Verification items for this drawing (mm, ordinates from the low corner). A direction names the side the tool comes from. Round coordinates to 2 decimals unless told otherwise and drop trailing zeros. Loops run counter-clockwise (first coordinate to the right, second up) from the corner with the lowest first, then second, coordinate; pieces in that order, holes last. Notation, with made-up numbers: (75.5, -27) - (121.5, -27) arc R28 cw to (121.5, -5) - close; hole circle Ø3 at (4.25, 19). An arc over 180 degrees is marked (long way). Put each result on its own line as item: value.
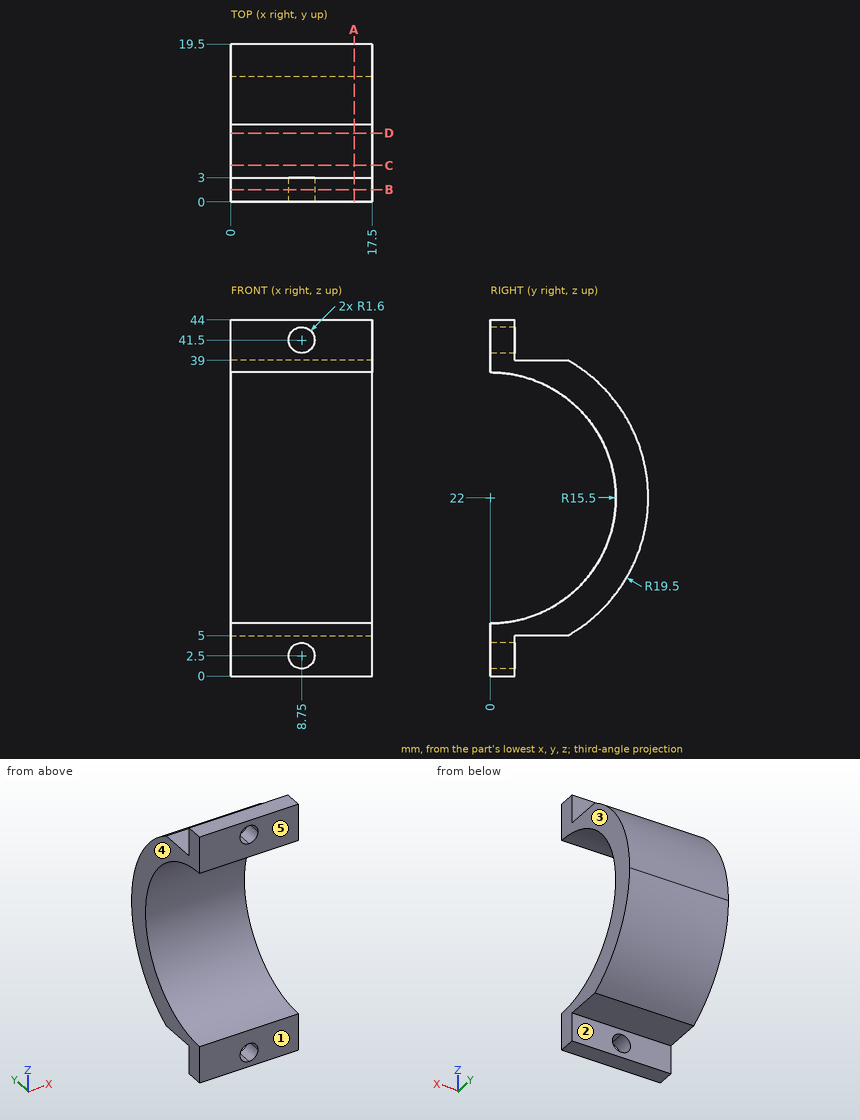
Item 1: Section check D-D on y = 8.5. Enter the section's corners in (x, z), then the cut area to 3 significant figures.
Filled sheet:
outline: (0, 5) - (17.5, 5) - (17.5, 9.04) - (0, 9.04) - close; (0, 34.96) - (17.5, 34.96) - (17.5, 39) - (0, 39) - close
area: 141 mm²
Item 2: Section check B-B on y = 1.5. Enter the section's corners in (x, z), then the cut area to 3 significant figures.
Filled sheet:
outline: (0, 0) - (17.5, 0) - (17.5, 6.57) - (0, 6.57) - close; (0, 37.43) - (17.5, 37.43) - (17.5, 44) - (0, 44) - close; hole circle Ø3.2 at (8.75, 2.5); hole circle Ø3.2 at (8.75, 41.5)
area: 214 mm²
Item 3: Thickness scan on line 1 (Y direction, x = 5, z = 4); line 2 (Z direction, x = 5.75, y = 3.5); line 3 (Y direction, x = 13, z = 22). Record the ranges inside material, lowest first. Write a range as from..to.
Filled sheet:
line 1: 0..3
line 2: 5..6.9, 37.1..39
line 3: 15.5..19.5
Item 4: Go/stop test with flat-tipped pins: pin 1 (2.5 mm diameter, centred on x = 10.5, z = 2, fed in from +Y); pin 2 (2 mm diameter, centred on x = 7, y = 14, fed in from -Z); pin 3 (5 mm diameter, centred on x = 10.5, y = 7, fed in from +Z). Record where each tip stops, or that it passes through.
Filled sheet:
pin 1: y = 3
pin 2: z = 7.47
pin 3: z = 39
Item 5: Section check A-A on x = 15.25. Enter the section's corners in (y, z), then the cut area to 3 significant figures.
Filled sheet:
outline: (0, 0) - (3, 0) - (3, 5) - (9.55, 5) arc R19.5 ccw to (9.55, 39) - (3, 39) - (3, 44) - (0, 44) - (0, 37.5) arc R15.5 cw to (0, 6.5) - close
area: 218 mm²
Item 6: Tool access check on the marked faces 1 and 2. Record the directions out of +Z, -Z, +X, -X, +Y, -Y that give a thin tool (end or side, any length) a straight path to the whole face; none if there is none.
Filled sheet:
face 1: +Z, -Z, +X, -X, -Y
face 2: -Z, +X, -X, +Y
Item 7: Release check for a two-part mould opening along X. For the marked faces 3, 4 and 5 record: +X half, -X half, draft (parallel to the pull), parting line (faces both ways), or undercut.
Filled sheet:
face 3: +X half
face 4: -X half
face 5: draft
Item 8: Section check C-C on y = 4.5. Enter the section's corners in (x, z).
Filled sheet:
outline: (0, 5) - (17.5, 5) - (17.5, 7.17) - (0, 7.17) - close; (0, 36.83) - (17.5, 36.83) - (17.5, 39) - (0, 39) - close
